```python
from build123d import *

# Parameters (mm, degrees)
SKETCH2_R           = 20.5
BOSS_EXTRUDE2_DEPTH = 30
SKETCH4_R           = 15.5
SKETCH4_R_2         = 12
CUT_EXTRUDE2_DEPTH  = 5
SKETCH6_R           = 3.1
CUT_EXTRUDE3_DEPTH  = 35.419562394
CUT_EXTRUDE4_DEPTH  = 8
CUT_EXTRUDE6_DEPTH  = 8


with BuildPart() as part:
    # Sketch2 → Boss-Extrude2 (new body)
    with BuildSketch(Plane(origin=(0, 0, 0), x_dir=(1, 0, 0), z_dir=(0, 1, 0))):
        with Locations(Location((0, 0, 0), (0, 0, 270))):
            Circle(SKETCH2_R)
    extrude(amount=BOSS_EXTRUDE2_DEPTH)

    # Sketch4 → Cut-Extrude2 (cut)
    with BuildSketch(Plane.XZ):
        with Locations(Location((0, 0, 0), (0, 0, 270))):
            Circle(SKETCH4_R)
        with Locations(Location((0, 0, 0), (0, 0, 270))):
            Circle(SKETCH4_R_2, mode=Mode.SUBTRACT)
    extrude(amount=-CUT_EXTRUDE2_DEPTH, mode=Mode.SUBTRACT)

    # Sketch5 → Cut-Revolve1 (revolve, cut)
    with BuildSketch(Plane.XY, mode=Mode.PRIVATE) as cut_revolve1_sk:
        Polygon((0, 0), (0, 11.447203031), (3.1, 11.447203031), (11.5, 0), align=None)
    revolve(cut_revolve1_sk.sketch.rotate(Axis((0, 0, 0), (0, 1, 0)), 90), axis=Axis((0, 0, 0), (0, 1, 0)), mode=Mode.SUBTRACT)

    # Sketch6 → Cut-Extrude3 (cut, through all)
    with BuildSketch(Plane.XZ.offset(-11.447203031)):
        with Locations(Location((0, 0, 0), (0, 0, 270))):
            Circle(SKETCH6_R)
    extrude(amount=-CUT_EXTRUDE3_DEPTH, mode=Mode.SUBTRACT)

    # Sketch8 → Cut-Extrude4 (cut)
    with BuildSketch(Plane.XY.offset(20.5)):
        Polygon((-5.25, 30), (5.25, 30), (5.25, 25), (8.25, 25), (8.25, 19.8), (-8.25, 19.8), (-8.25, 25), (-5.25, 25), align=None)
    extrude(amount=-CUT_EXTRUDE4_DEPTH, mode=Mode.SUBTRACT)

    # Sketch9 → Cut-Extrude6 (cut)
    with BuildSketch(Plane.XY.offset(-20.5)):
        Polygon((5.25, 30), (-5.25, 30), (-5.25, 25), (-8.25, 25), (-8.25, 19.8), (8.25, 19.8), (8.25, 25), (5.25, 25), align=None)
    extrude(amount=CUT_EXTRUDE6_DEPTH, mode=Mode.SUBTRACT)


solid = part.part
```
Can you work these out from the model? Positions are in its coordinate system, mm. A direction names the side the tool comes from. Give positions to 0.01 mm unless a question says otherwise; leave off trailing zeros. Order: outer loops, then holes, each group sorted by start corner. A loop starts at its lowest first (then second) coordinate and runs counter-clockwise, first axis right, second up. Notation, with made-up numbers: M -5.5,-24 L 40.5,-24 A18 cw 40.5,-5 Z; hole C 58.5,-36.75 d2. An arc over 180 degrees is marked long. Write item = value, one per line. Start each with the question number.
Q1. I need wall thicknesses on probe 1 along Y at (x, z) = (5.5, -18); probe 2 along X at (y, z) = (17.75, 0); probe 3 along X at (y, z) = (2.8, 0). Which ranges of each line are inside material? Lowest first, please. Write a range as [from, to].
Q2. Suppose I cut it at A-A (x = 0). Write out the boundary of the cut face in (y, z).
Q3. Suppose I cut it at B-B (z = 0). Write out the boundary of the cut face in (x, y), plus the area to 3 significant figures.
Q4. For faces 5 (the flat face through (-5.25, 28, -16)), 6 (the flat face through (7, 25, -16)), 7 (the flat face through (-5.25, 27, 16)), 8 (the flat face through (0, 19.8, 17)), 9 (the cylindrical face through (3.604, 2.465, -11.446)), which set-ups out of +Z, -Z, +X, -X, +Y, -Y let a thin tool reach every point of the face, with its end or its side?
Q5. Will these pins go through, and if not, where does the flat tip stop? pin 1 Ø10 at (y, z) = (26, 9.5) entering from -X; pin 2 Ø5.5 at (y, z) = (26.5, -16) entering from +X; pin 3 Ø2 at (x, y) = (-0.5, 19) entering from -Z; pin 4 Ø8 at (x, y) = (-3, 23) entering from +Z.
Q6. Suppose I cut it at C-C (y = 21.5). Write out the boundary of the cut face in (x, z).
Q7. Suppose I cut it at D-D (y = 3). Write out the boundary of the cut face in (x, z).
Q8. We'd pull the mould along Y, two halves only. Please class faces 1 (the flat face through (-11.4, 5, -4.5)), 2 (the flat face through (-4, 30, 0)), 3 (the cylindrical face through (15.368, 2.465, 2.018)), 4 (the flat face through (8.25, 22, 16)): pulls with the +Y half, pulls with the -Y half, needs draft (parallel to the pull), parting line crosses it, or undercut.
Check result:
q1.probe_1 = [0, 19.8], [25, 30]
q1.probe_2 = [-20.5, -3.1], [3.1, 20.5]
q1.probe_3 = [-20.5, -15.5], [-12, -9.45], [9.45, 12], [15.5, 20.5]
q2.outline = M 0,-20.5 L 19.8,-20.5 L 19.8,-12.5 L 30,-12.5 L 30,-3.1 L 11.45,-3.1 L 0,-11.5 L 0,-12 L 5,-12 L 5,-15.5 L 0,-15.5 Z; M 0,11.5 L 11.45,3.1 L 30,3.1 L 30,12.5 L 19.8,12.5 L 19.8,20.5 L 0,20.5 L 0,15.5 L 5,15.5 L 5,12 L 0,12 Z
q3.outline = M -20.5,0 L -15.5,0 L -15.5,5 L -12,5 L -12,0 L -11.5,0 L -3.1,11.45 L -3.1,30 L -20.5,30 Z; M 3.1,11.45 L 11.5,0 L 12,0 L 12,5 L 15.5,5 L 15.5,0 L 20.5,0 L 20.5,30 L 3.1,30 Z
q3.area = 913 mm2
q4.face_5 = -Z, +Y
q4.face_6 = -Z
q4.face_7 = +Z, +Y
q4.face_8 = +Z
q4.face_9 = -Y
q5.pin_1 = -20
q5.pin_2 = 15.64
q5.pin_3 = -20.5
q5.pin_4 = 20.49
q6.outline = M -8.25,-18.77 L -8.25,-12.5 L 8.25,-12.5 L 8.25,-18.77 A20.5 ccw 8.25,18.77 L 8.25,12.5 L -8.25,12.5 L -8.25,18.77 A20.5 ccw Z; hole C 0,0 d6.2
q7.outline = C 0,0 d41; C 0,0 d24; hole C 0,0 d31; hole C 0,0 d18.6
q8.face_1 = pulls with the -Y half
q8.face_2 = pulls with the +Y half
q8.face_3 = needs draft
q8.face_4 = undercut
